Here's how the part is built. I have some questions about the finished solid (model axes, mm). Face numbers are marked on the shaded views. A direction names the side the tool comes from. Give positions to 0.01 mm unless a question says otherwise; leave off trailing zeros. Write each loop counter-clockwise with the first axis right and the second up, starting at its lowest first coordinate (ties: lowest second). Pieces come first, ordered by that corner, then holes. Notation, with made-up numbers: (30.25, 45.25) - (56.25, 45.25) arc R33 cw to (56.25, 76.25) - close; hole circle Ø2 at (16, 57.5). An arc over 180 degrees is marked (long way). One line per item, written item: value. Start each with the question number.
1) I'm going to push flat-ended pins straight in: P1, Ø3, axis at x = -20.5, z = 245.5, coming from the +Y side; P2, Ø4, axis at y = -9.5, z = 196.5, coming from the +X side; P3, Ø15.5, axis at y = 3.5, z = 245, coming from the -X side. Where does each tip first touch, or does it pass through?
2) Imagine slicing it at A-A on x = 0. Write out the boundary of the cut face in (y, z), plus the area to 3 significant figures.
3) Please list where these lines run through material, in increasing order: L1, parallel to Z at x = 23, y = 3.5; L2, parallel to Z at x = -14.5, y = -1.5; L3, parallel to Y at x = 22.5, z = -207. Write a range as [from, to].
4) On a 3-axis mill with a long thin cutter (end or side, diameter ignored), from which of +Z, -Z, +X, -X, +Y, -Y can I reach the whole of each face in a straight line? I mean the marked faces 1 and 2. Say none if no direction works.
5) Imagine slicing it at D-D on z = -142.5. Write out the boundary of the cut face in (x, y).
6) Imagine slicing it at B-B on y = 0. Write out the boundary of the cut face in (x, z), plus the area to 3 significant figures.
7) Imagine slicing it at C-C on z = 179. Write out the boundary of the cut face in (x, y), plus the area to 3 significant figures.
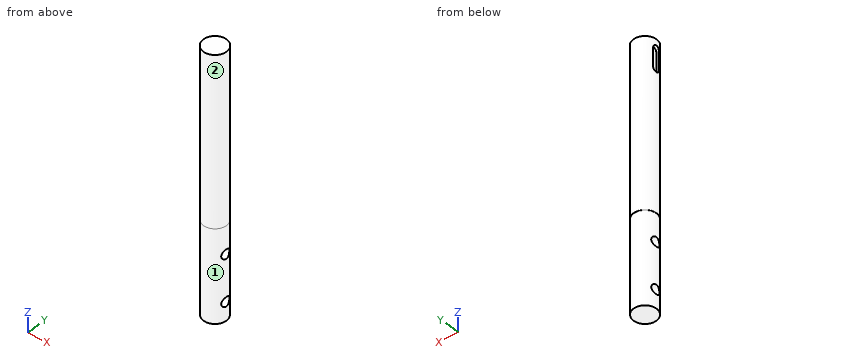
from build123d import *

# Parameters (mm, degrees)
SKETCH1_R               = 25
BOSS_EXTRUDE1_DEPTH     = 282.5
CUT_EXTRUDE1_DEPTH      = 285.703793442
CUT_EXTRUDE1_DEPTH_BACK = 285.703793442
SKETCH2_R               = 10.05
CUT_EXTRUDE2_DEPTH      = 10
SKETCH4_OUTSIDE_W       = 165.882
SKETCH4_OUTSIDE_H       = 165.882
SKETCH4_OUTSIDE_R       = 24.61
CUT_EXTRUDE3_DEPTH      = 200


with BuildPart() as part:
    # Sketch1 → Boss-Extrude1 (new, symmetric)
    with BuildSketch(Plane.XY):
        Circle(SKETCH1_R)
    extrude(amount=BOSS_EXTRUDE1_DEPTH, both=True)

    # Sketch2 → Cut-Extrude1 (cut, two sides: drawn at the far end of the back side and taken through both)
    with BuildSketch(Plane(origin=(0, 0, 0), x_dir=(0, 0, -1), z_dir=(1, 0, 0)).offset(-CUT_EXTRUDE1_DEPTH_BACK)):
        with Locations(Location((142.5, 0, 0), (0, 0, 180))):
            Circle(SKETCH2_R)
        with Locations(Location((242.5, 0, 0), (0, 0, 180))):
            Circle(SKETCH2_R)
    extrude(amount=CUT_EXTRUDE1_DEPTH + CUT_EXTRUDE1_DEPTH_BACK, mode=Mode.SUBTRACT)

    # Sketch3 → Cut-Extrude2 (cut)
    with BuildSketch(Plane(origin=(-18.5, 0, 0), x_dir=(0, 0, -1), z_dir=(1, 0, 0))):
        with BuildLine():
            Line((-262.5, -7), (-220.5, -7))
            ThreePointArc((-220.5, -7), (-213.5, 0), (-220.5, 7))
            Line((-220.5, 7), (-262.5, 7))
            ThreePointArc((-262.5, 7), (-269.5, 0), (-262.5, -7))
        make_face()
    extrude(amount=-CUT_EXTRUDE2_DEPTH, mode=Mode.SUBTRACT)

    # Sketch4 outside → Cut-Extrude3 (cut)
    with BuildSketch(Plane(origin=(0, 0, -282.5), x_dir=(-1, 0, 0), z_dir=(0, 0, -1))):
        Rectangle(SKETCH4_OUTSIDE_W, SKETCH4_OUTSIDE_H)
        Circle(SKETCH4_OUTSIDE_R, mode=Mode.SUBTRACT)
    extrude(amount=-CUT_EXTRUDE3_DEPTH, mode=Mode.SUBTRACT)


solid = part.part
Numbers:
1. P1: y = 16.25
1. P2: x = 23.85
1. P3: x = -24
2. outline: (-25, -82.5) - (-24.61, -82.5) - (-24.61, -282.5) - (24.61, -282.5) - (24.61, -82.5) - (25, -82.5) - (25, 282.5) - (-25, 282.5) - close; hole circle Ø20.1 at (0, -242.5); hole circle Ø20.1 at (0, -142.5)
2. area: 27,500 mm^2
3. L1: [-282.5, -251.92], [-233.08, -151.92], [-133.08, 282.5]
3. L2: [-282.5, -252.44], [-232.56, -152.44], [-132.56, 282.5]
3. L3: [-9.97, 9.97]
4. face 1: -Z
4. face 2: +Z, -Z
5. outline: (-22.46, -10.05) arc R24.61 ccw to (22.46, -10.05) - close; (-22.46, 10.05) - (22.46, 10.05) arc R24.61 ccw to start
6. outline: (-25, -82.5) - (-24.61, -82.5) - (-24.61, -132.45) - (24.61, -132.45) - (24.61, -82.5) - (25, -82.5) - (25, 282.5) - (-25, 282.5) - (-25, 269.5) - (-18.5, 269.5) - (-18.5, 213.5) - (-25, 213.5) - close; (-24.61, -282.5) - (24.61, -282.5) - (24.61, -252.55) - (-24.61, -252.55) - close; (-24.61, -232.45) - (24.61, -232.45) - (24.61, -152.55) - (-24.61, -152.55) - close
6. area: 25,800 mm^2
7. outline: circle Ø50 at (0, 0)
7. area: 1,960 mm^2
